Autodesk Inventor part; units mm, degrees
ref_plane "YZ Plane" through (0, 0, 0) normal (1, 0, 0) x (0, 1, 0)
ref_plane "XZ Plane" through (0, 0, 0) normal (0, 1, 0) x (-1, 0, 0)
ref_plane "XY Plane" through (0, 0, 0) normal (0, 0, 1) x (1, 0, 0)
sketch "Sketch1" plane through (0, 0, 0) normal (0, 0, 1) x (1, 0, 0)
  circle A0 centre (0, 0) radius 26.5
  dimension "d0" = 53
extrude "Extrusion1" add sketch "Sketch1" along normal blind 0.2
sketch "Sketch2" plane through (0, 0, 0.2) normal (0, 0, 1) x (1, 0, 0)
  circle A0 centre (0, 0) radius 23 construction
  point P0 (23, 0)
  dimension "d3" = 46
hole "Hole1" at (23, 0, 0.2) direction (0, 0, -1) diameter 3.2 end through all
pattern_circular "Circular Pattern1" count 4 over 360 about axis through (0, 0, 0) along (0, 0, 1) of "Hole1"
properties part number "probe-gate-mesh-circle-53mm" material "Stainless Steel"
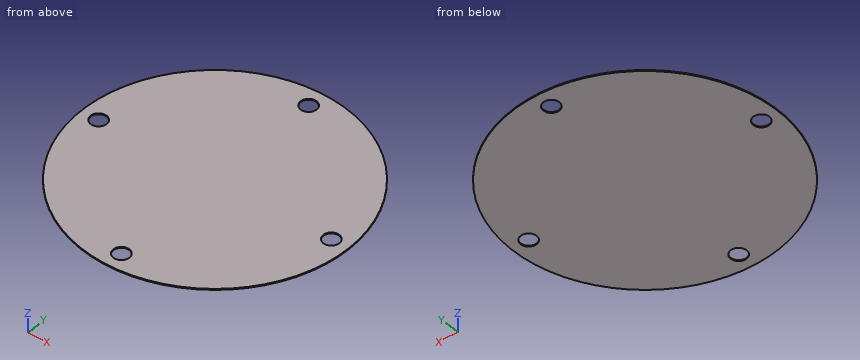
The listing builds one solid part. Answer for the finished solid, in the listing's coordinates (mm). Round coordinates to 2 decimals unless told otherwise and drop trailing zeros. Loops run counter-clockwise (first coordinate to the right, second up) from the corner with the lowest first, then second, coordinate; pieces in that order, holes last. Notation, with made-up numbers: M -19.5,42.5 L 27.5,42.5 A15 ccw 27.5,71.5 Z; hole C -31.5,-36.75 d5. An arc over 180 degrees is marked long. Write each question's results on one line, items separated by ' | '. Start each with the question number.
1) Find section D-D on z = 0.15. Write down the section's boundary in (x, y).
2) Find section A-A on y = 0. Write down the section's boundary in (x, z), plus the area to 3 significant figures.
3) Straight lines are drawn through the part: probe 1 along Y at (x, z) = (0, 0.05); probe 2 along Y at (x, z) = (-1, 0.15); probe 3 along X at (y, z) = (23, 0.15). For each, find the intervals that lie inside material, in ascending order.
4) Find section C-C on x = 23. Write down the section's boundary in (y, z), plus the area to 3 significant figures.
5) Each of these flat-tipped pins is pushed along its axis until it touches: pin 1 (1.9 mm diameter, centred on x = 0, y = -23, fed in from +Z); pin 2 (10 mm diameter, centred on x = 15, y = 11, fed in from -Z). Where does it stop, or does it pass through?
Final values:
1) outline: C 0,0 d53; hole C -23,0 d3.2; hole C 0,-23 d3.2; hole C 0,23 d3.2; hole C 23,0 d3.2
2) outline: M -26.5,0 L -24.6,0 L -24.6,0.2 L -26.5,0.2 Z; M -21.4,0 L 21.4,0 L 21.4,0.2 L -21.4,0.2 Z; M 24.6,0 L 26.5,0 L 26.5,0.2 L 24.6,0.2 Z | area: 9.32 mm²
3) probe 1: -26.5 to -24.6, -21.4 to 21.4, 24.6 to 26.5 | probe 2: -26.48 to -24.25, -21.75 to 21.75, 24.25 to 26.48 | probe 3: -13.16 to -1.6, 1.6 to 13.16
4) outline: M -13.16,0 L -1.6,0 L -1.6,0.2 L -13.16,0.2 Z; M 1.6,0 L 13.16,0 L 13.16,0.2 L 1.6,0.2 Z | area: 4.62 mm²
5) pin 1: through | pin 2: z = 0
